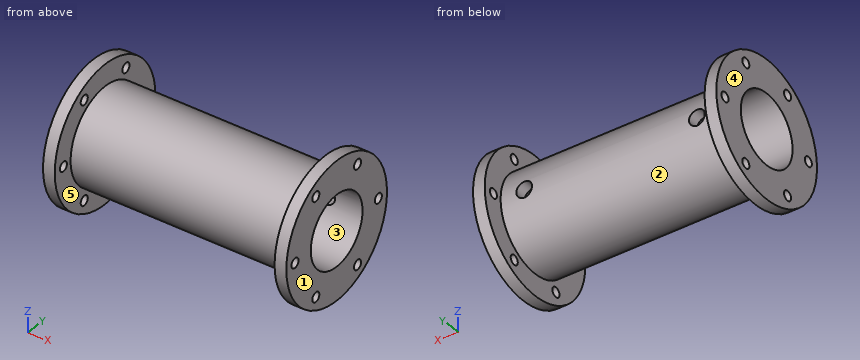
Autodesk Inventor part; units mm, degrees
ref_plane "Work Plane1" through (31, 0, 0) normal (1, 0, 0) x (0, 0, -1)
ref_plane "Work Plane3" through (0, 12, 0) normal (0, 1, 0) x (-1, 0, 0)
ref_plane "YZ Plane" through (0, 0, 0) normal (1, 0, 0) x (0, 1, 0)
sketch "Sketch1" plane through (0, 0, 0) normal (0, 0, 1) x (1, 0, 0)
  line L0 (-31, 0) -> (-31, 17.5)
  line L1 (-31, 17.5) -> (-28, 17.5)
  line L2 (-28, 17.5) -> (-28, 12)
  line L3 (-28, 12) -> (28, 12)
  line L4 (28, 12) -> (28, 17.5)
  line L5 (28, 17.5) -> (31, 17.5)
  line L6 (31, 17.5) -> (31, 0)
  line L7 (31, 0) -> (-31, 0)
  point P0 (0, 0)
  point P1 (0, 0)
  dimension "d0" = 24
  dimension "d1" = 35
  dimension "d2" = 3
  dimension "d3" = 3
  dimension "d4" = 56
revolve "Revolution1" add sketch "Sketch1" angle 360 about axis through (31, 0, 0) along (-1, 0, 0)
sketch "Sketch2" plane through (31, 0, 0) normal (1, 0, 0) x (0, 0, -1)
  circle A0 centre (0, 0) radius 17.5
  point P0 (0, 0)
hole "Hole1" at (31, 0, 0) direction (-1, 0, 0) diameter 18 end through all
ref_plane "Work Plane1" through (31, 0, 0) normal (1, 0, 0) x (0, 0, -1)
sketch "Sketch3" plane through (31, 0, 0) normal (1, 0, 0) x (0, 0, -1)
  line L0 (0, 0) -> (-20.6833, 0) construction
  line L1 (0, 0) -> (-12.5574, -7.25) construction
  circle A0 centre (0, 0) radius 14.5 construction
  dimension "d15" = 29
  dimension "d14" = 30
hole "Hole2" at (31, -7.25, 12.5574) direction (-1, 0, 0) diameter 2.459 depth 3
pattern_circular "Circular Pattern1" count 6 over 360 about axis through (29.5, 0, 0) along (-1, 0, 0) of "Hole2"
mirror "Mirror1" about plane through (0, 0, 0) normal (1, 0, 0) of "Hole2", "Circular Pattern1"
ref_plane "Work Plane3" through (0, 12, 0) normal (0, 1, 0) x (-1, 0, 0)
sketch "Sketch5" plane through (0, 12, 0) normal (0, 1, 0) x (-1, 0, 0)
  line L0 (28, -17.5) -> (28, 17.5)
  line L1 (-28, -17.5) -> (-28, 17.5)
  point P0 (0, 0)
  point P1 (22, 0)
  point P2 (-22, 0)
  dimension "d37" = 6
  dimension "d38" = 6
hole "Hole4" at (-22, 12, 0) at (22, 12, 0) direction (0, -1, 0) diameter 4 depth 3.5
properties part number "154" material "Stainless Steel"
The listing builds one solid part. Answer for the finished solid, in the listing's coordinates (mm). Face numbers are marked on the shaded views. A direction names the side the tool comes from. Coordinates: 2 decimals unless noted, no trailing zeros. Write each loop counter-clockwise with the first axis right and the second up, starting at its lowest first coordinate (ties: lowest second). Pieces come first, ordered by that corner, then holes. Notation, with made-up numbers: M 16.25,31.25 L 42.25,31.25 A10 ccw 42.25,40.25 Z; hole C -29,-22 d5. An arc over 180 degrees is marked long. Use a Markdown table: item, result. Add a question column.
1. Section C-C (y = 7.25) is taken. Count the separate pieces of the cut face and the enclosed holes in it, plus the area to 3 significant figures.
2. Straight lines are drawn through the part: line 1 along X through (y, z) = (9.75, 0); line 2 along X through (y, z) = (-14.5, 9); line 3 along Y through (x, z) = (10.5, 0). For each, find the intervals that lie inside material, in ascending order. Write a range as [from, to].
3. Which of the six approach directions +Z, -Z, +X, -X, +Y, -Y give full straight-line access (tool end or side, diameter ignored) to the marked faces 4 and 5?
4. For a pull along Z with two mould halves and no side action, classify the marked faces 1, 2 and 3 as +Z half, -Z half, draft (parallel to the pull), parting line (faces both ways), or undercut.
5. Section B-B (z = -7.5) is taken. Give the vertices of the cut face in (x, y).
6. Section D-D (z = 15) is taken. Give the vertices of the cut face in (x, y).
7. Section A-A (y = 0) is taken. Give the vertices of the cut face in (x, z), plus the area to 3 significant figures.
8. Given P1, Ø2, axis at y = 7.25, z = 12.56, coming from the +X side; P2, Ø4, axis at x = -9, z = -6, coming from the -Y side; P3, Ø2, axis at x = 20.5, y = 11.5, coming from the +Z side; P4, Ø6, axis at x = -7.5, y = 2.5, coming from the +Z side, each flat-ended and moving along its own axis, determine where each tip first touches the part or whether it passes through.
Data:
| question | item | result |
|---|---|---|
| 1 | separate pieces | 6 |
| 1 | enclosed holes | 0 |
| 1 | area | 571 mm2 |
| 2 | line 1 | x = [-31, -24], [-20, 20], [24, 31] |
| 2 | line 2 | x = [-31, -28], [28, 31] |
| 2 | line 3 | y = [-12, -9], [9, 12] |
| 3 | face 4 | +Z, -Z, -X, +Y, -Y |
| 3 | face 5 | none |
| 4 | face 1 | draft |
| 4 | face 2 | parting line |
| 4 | face 3 | undercut |
| 5 | outline | M -31,-15.81 L -28,-15.81 L -28,-9.37 L 28,-9.37 L 28,-15.81 L 31,-15.81 L 31,-4.97 L -31,-4.97 Z; M -31,4.97 L 31,4.97 L 31,15.81 L 28,15.81 L 28,9.37 L -28,9.37 L -28,15.81 L -31,15.81 Z |
| 6 | outline | M -31,-9.01 L -28,-9.01 L -28,9.01 L -31,9.01 Z; M 28,-9.01 L 31,-9.01 L 31,9.01 L 28,9.01 Z |
| 7 | outline | M -31,-17.5 L -28,-17.5 L -28,-12 L 28,-12 L 28,-17.5 L 31,-17.5 L 31,-9 L -31,-9 Z; M -31,9 L 31,9 L 31,17.5 L 28,17.5 L 28,12 L -28,12 L -28,17.5 L -31,17.5 Z |
| 7 | area | 438 mm2 |
| 8 | P1 | passes through |
| 8 | P2 | stops at y = -11.31 |
| 8 | P3 | stops at z = 5.81 |
| 8 | P4 | stops at z = 12 |
